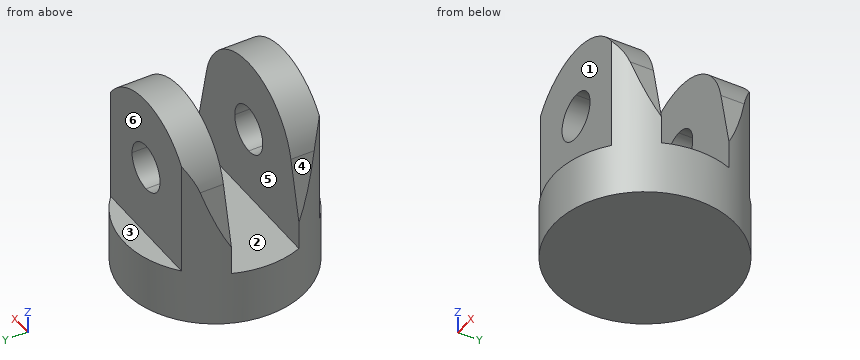
from build123d import *

# Parameters (mm, degrees)
F0_R     = 12.7
F1_DEPTH = 7.62
F3_DEPTH = 12.7
F4_W     = 3.0988
F4_H     = 21.7537892061
F4_H_2   = 20.3239873993
F5_DEPTH = 12.7
F6_DEPTH = 12.7
F7_DEPTH = 25.4
F8_DEPTH = 12.7


with BuildPart() as f1:
    # F0 (on Top) → F1 (new body)
    with BuildSketch(Plane.XY):
        Circle(F0_R)
    extrude(amount=F1_DEPTH)

    # F2 (on Front) → F3 (cut, symmetric)
    with BuildSketch(Plane.XZ):
        with BuildLine():
            ThreePointArc((0, 21.0693), (-3.2893, 17.78), (0, 14.4907))
            Line((0, 14.4907), (0, 21.0693))
        make_face()
        with BuildLine():
            Line((0, 21.0693), (0, 14.4907))
            ThreePointArc((0, 14.4907), (2.3258863354, 15.4541136646), (3.2893, 17.78))
            ThreePointArc((3.2893, 17.78), (2.3258863354, 20.1058863354), (0, 21.0693))
        make_face()
    extrude(amount=F3_DEPTH, both=True, mode=Mode.SUBTRACT)

    # F4 (on Right) → F5 (cut, symmetric)
    with BuildSketch(Plane.YZ):
        with Locations((11.1506, 18.4968946031)):
            Rectangle(F4_W, F4_H)
        Polygon((-4.699, 7.62), (0, 7.62), (4.699, 7.62), (4.699, 28.9018824697), (0, 28.9018824697), (-4.699, 28.9018824697), (-4.699, 27.9439873993), align=None)
        with Locations((-11.1506, 17.7819936997)):
            Rectangle(F4_W, F4_H_2)
    extrude(amount=F5_DEPTH, both=True, mode=Mode.SUBTRACT)

    # F2 (on Front) → F6 (join, symmetric)
    with BuildSketch(Plane.XZ):
        with BuildLine():
            ThreePointArc((0, 7.62), (7.1842048969, 10.5957951031), (10.16, 17.78))
            ThreePointArc((10.16, 17.78), (10.0978587443, 18.9019843049), (9.912195122, 20.0102439024))
            ThreePointArc((9.912195122, 20.0102439024), (6.3469016832, 25.7136271039), (0, 27.94))
            Line((0, 27.94), (0, 21.0693))
            ThreePointArc((0, 21.0693), (2.3258863354, 20.1058863354), (3.2893, 17.78))
            ThreePointArc((3.2893, 17.78), (2.3258863354, 15.4541136646), (0, 14.4907))
            Line((0, 14.4907), (0, 7.62))
        make_face()
        with BuildLine():
            ThreePointArc((9.912195122, 20.0102439024), (10.0978587443, 18.9019843049), (10.16, 17.78))
            ThreePointArc((10.16, 17.78), (7.1842048969, 10.5957951031), (0, 7.62))
            Line((0, 7.62), (12.7, 7.62))
            Line((12.7, 7.62), (9.912195122, 20.0102439024))
        make_face()
        with BuildLine():
            Line((-12.7, 7.62), (0, 7.62))
            ThreePointArc((0, 7.62), (-7.9336271039, 11.4330983168), (-9.912195122, 20.0102439024))
            Line((-9.912195122, 20.0102439024), (-12.7, 7.62))
        make_face()
        with BuildLine():
            ThreePointArc((-9.912195122, 20.0102439024), (-7.9336271039, 11.4330983168), (0, 7.62))
            Line((0, 7.62), (0, 14.4907))
            ThreePointArc((0, 14.4907), (-3.2893, 17.78), (0, 21.0693))
            Line((0, 21.0693), (0, 27.94))
            ThreePointArc((0, 27.94), (-6.3469016832, 25.7136271039), (-9.912195122, 20.0102439024))
        make_face()
    extrude(amount=F6_DEPTH, both=True)

    # F7 (cut): faces of the model
    f7_faces = [f1.faces().sort_by_distance(p)[0] for p in [
        (-9.8632271754, 9.8632271754, 7.62),
        (9.8632271754, 9.8632271754, 7.62),
        (9.8632271754, -9.8632271754, 7.62),
        (-9.8632271754, -9.8632271754, 7.62),
    ]]
    extrude(f7_faces, amount=-F7_DEPTH, mode=Mode.SUBTRACT)

    # F4 (on Right) → F8 (cut, symmetric)
    with BuildSketch(Plane.YZ):
        with Locations((11.1506, 18.4968946031)):
            Rectangle(F4_W, F4_H)
        Polygon((-4.699, 7.62), (0, 7.62), (4.699, 7.62), (4.699, 28.9018824697), (0, 28.9018824697), (-4.699, 28.9018824697), (-4.699, 27.9439873993), align=None)
        with Locations((-11.1506, 17.7819936997)):
            Rectangle(F4_W, F4_H_2)
    extrude(amount=F8_DEPTH, both=True, mode=Mode.SUBTRACT)


solid = f1.part
Design review of the part built by this model. Coordinates are the model's own, in mm. Face numbers are marked on the shaded views. A direction names the side the tool comes from. Give positions to 0.01 mm unless a question says otherwise; leave off trailing zeros. Loops run counter-clockwise (first coordinate to the right, second up) from the corner with the lowest first, then second, coordinate; pieces in that order, holes last. Notation, with made-up numbers: M 32,48 L 68,48 A26 cw 68,82 Z; hole C 48.25,-39 d3. An arc over 180 degrees is marked long. Answer as a JSON object with one key per item and string values.
Item 1: We need section B-B (z = 12.25). State the section outline as (x, y) points, and give its area (3 significant figures).
Output values:
{"outline": "M -11.66,-5.04 A12.7 ccw -8.31,-9.6 L 8.31,-9.6 A12.7 ccw 11.66,-5.04 L 11.66,-4.7 L -11.66,-4.7 Z; M -11.66,4.7 L 11.66,4.7 L 11.66,5.04 A12.7 ccw 8.31,9.6 L -8.31,9.6 A12.7 ccw -11.66,5.04 Z", "area": "203 mm2"}
Item 2: For P1, Ø1, axis at x = 0.5, y = 1.5, coming from the +Z side; P2, Ø3, axis at x = -2, y = -4, coming from the +Z side; P3, Ø10, axis at x = 4, z = 13, coming from the -Y side, all flat-tipped, find the tip position at first contact; note any pin that passes through.
Output values:
{"P1": "stops at z = 7.62", "P2": "stops at z = 27.92", "P3": "stops at y = -9.6"}
Item 3: Wall thickness on line 1 along Y through (x, z) = (5.25, 23); line 2 along Z through (x, y) = (-4.25, 3.5); line 3 along X through (y, z) = (7, 19): over which ranges is each line inside the solid? List them lowest first.
Output values:
{"line 1": "y = -9.6 to -4.7, 4.7 to 9.6", "line 2": "z = 0 to 7.62", "line 3": "x = -10.14 to -3.05, 3.05 to 10.14"}
Item 4: We need section C-C (y = -5.5). State the section outline as (x, z) points.
Output values:
{"outline": "M -11.45,0 L 11.45,0 L 11.45,13.19 L 9.91,20.01 A10.16 ccw -9.91,20.01 L -11.45,13.19 Z; hole C 0,17.78 d6.58"}
Item 5: Machinability: for the marked faces 1, 2 and 3, which of the approach directions +Z, -Z, +X, -X, +Y, -Y give a long, thin tool a straight path to every point of the face, cutting with its end or side? Answer none if there is none.
Output values:
{"face 1": "+Z, +X, -X, -Y", "face 2": "+Z, +X, -X", "face 3": "+Z, +X, -X, +Y"}
Item 6: We need section D-D (x = -9). State the section outline as (y, z) points.
Output values:
{"outline": "M -8.96,0 L 8.96,0 L 8.96,22.49 L 4.7,22.49 L 4.7,7.62 L -4.7,7.62 L -4.7,22.49 L -8.96,22.49 Z"}
Item 7: Mouldability with a two-part tool opening along Y and no side actions: class the marked faces 4, 5 and 6 as pulls with the +Y half, pulls with the -Y half, needs draft (parallel to the pull), parting line crosses it, or undercut.
Output values:
{"face 4": "needs draft", "face 5": "undercut", "face 6": "pulls with the +Y half"}
Item 8: We need section A-A (x = -0.5). State the section outline as (y, z) points.
Output values:
{"outline": "M -12.69,0 L 12.69,0 L 12.69,7.62 L 9.6,7.62 L 9.6,14.53 L 4.7,14.53 L 4.7,7.62 L -4.7,7.62 L -4.7,14.53 L -9.6,14.53 L -9.6,7.62 L -12.69,7.62 Z; M -9.6,21.03 L -4.7,21.03 L -4.7,27.93 L -9.6,27.93 Z; M 4.7,21.03 L 9.6,21.03 L 9.6,27.93 L 4.7,27.93 Z"}
